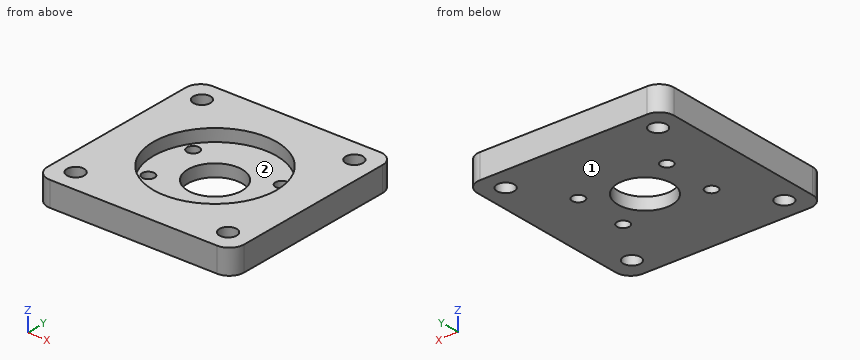
```python
from build123d import *

# Parameters (mm, degrees)
F0_W     = 40
F0_H     = 40
F0_R     = 1.75
F0_R_2   = 1.25
F0_R_3   = 5.5
F1_DEPTH = 5
F2_R     = 12.5
F3_DEPTH = 2.5
F4_R     = 3


with BuildPart() as f1:
    # F0 (on Top) → F1 (new body)
    with BuildSketch(Plane.XY):
        Rectangle(F0_W, F0_H)
        with Locations((-15.5, -15.5)):
            Circle(F0_R, mode=Mode.SUBTRACT)
        with Locations((-9, -5.5)):
            Circle(F0_R_2, mode=Mode.SUBTRACT)
        with Locations((15.5, -15.5)):
            Circle(F0_R, mode=Mode.SUBTRACT)
        with Locations((9, -5.5)):
            Circle(F0_R_2, mode=Mode.SUBTRACT)
        with Locations((-9, 5.5)):
            Circle(F0_R_2, mode=Mode.SUBTRACT)
        with Locations((-15.5, 15.5)):
            Circle(F0_R, mode=Mode.SUBTRACT)
        Circle(F0_R_3, mode=Mode.SUBTRACT)
        with Locations((9, 5.5)):
            Circle(F0_R_2, mode=Mode.SUBTRACT)
        with Locations((15.5, 15.5)):
            Circle(F0_R, mode=Mode.SUBTRACT)
    extrude(amount=F1_DEPTH)

    # F2 (on face) → F3 (cut)
    with BuildSketch(Plane.XY.offset(5)):
        Circle(F2_R)
    extrude(amount=-F3_DEPTH, mode=Mode.SUBTRACT)

    # F4
    f4_edges = [f1.edges().sort_by_distance(p)[0] for p in [
        (-20, -20, 2.5),
        (20, -20, 2.5),
        (20, 20, 2.5),
        (-20, 20, 2.5),
    ]]
    fillet(f4_edges, radius=F4_R)


solid = f1.part
```
Geometry: final body of the model. Coordinates: model frame, mm. Face numbers are marked on the shaded views. A direction names the side the tool comes from. Round coordinates to 2 decimals unless told otherwise and drop trailing zeros. Loops run counter-clockwise (first coordinate to the right, second up) from the corner with the lowest first, then second, coordinate; pieces in that order, holes last.
Item 1: Section D-D, the plane y = 0. Output: boundary loops of the cut face in (x, z), plus the area to 3 significant figures.
Checked values:
outline: (-20, 0) - (-5.5, 0) - (-5.5, 2.5) - (-12.5, 2.5) - (-12.5, 5) - (-20, 5) - close; (5.5, 0) - (20, 0) - (20, 5) - (12.5, 5) - (12.5, 2.5) - (5.5, 2.5) - close
area: 110 mm2
Item 2: Contact query for flat-ended pins moving along their axis: P1, Ø4, axis at x = 9, y = -5.5, coming from the -Z side; P2, Ø12.5, axis at x = 0, y = -5.5, coming from the +Z side. Output: stop coordinate, or through.
Checked values:
P1: stops at z = 0
P2: stops at z = 2.5
Item 3: Line query: L1, parallel to Y at x = 9, z = 1.95; L2, parallel to X at y = -0.5, z = 2.9; L3, parallel to Y at x = -15.5, z = 1.05. Output: solid intervals per line, ascending.
Checked values:
L1: y = -20 to -6.75, -4.25 to 4.25, 6.75 to 20
L2: x = -20 to -12.49, 12.49 to 20
L3: y = -20 to -17.25, -13.75 to 13.75, 17.25 to 20
Item 4: Reachability of the marked faces 1 and 2 from +Z, -Z, +X, -X, +Y, -Y: full face, straight path, thin tool, end or side. Return the list, or none.
Checked values:
face 1: -Z, +X, -X, +Y, -Y
face 2: +Z
Item 5: Section A-A, the plane x = -15.5. Output: boundary loops of the cut face in (y, z), plus the area to 3 significant figures.
Checked values:
outline: (-20, 0) - (-17.25, 0) - (-17.25, 5) - (-20, 5) - close; (-13.75, 0) - (13.75, 0) - (13.75, 5) - (-13.75, 5) - close; (17.25, 0) - (20, 0) - (20, 5) - (17.25, 5) - close
area: 165 mm2
Item 6: Section C-C, the plane z = 0.8. State how many separate pieces and enclosed holes the cut face has, plus the area to 3 significant figures.
Checked values:
separate pieces: 1
enclosed holes: 9
area: 1,440 mm2
